from build123d import *

# Parameters (mm, degrees)
SKETCH_1_R           = 23
EXTRUDE_1_DEPTH      = 6
EXTRUDE_2_DEPTH      = 25
EXTRUDE_2_DEPTH_BACK = 9
SKETCH_2_R           = 18
SKETCH_3_R           = 10.25
CUT_EXTRUDE_1_DEPTH  = 48.053161424


with BuildPart() as part:
    # 草图1 → 凸台-拉伸1 (new body)
    with BuildSketch(Plane(origin=(0, 0, 0), x_dir=(0, 0, -1), z_dir=(1, 0, 0))):
        Circle(SKETCH_1_R)
    extrude(amount=EXTRUDE_1_DEPTH)

    # 草图2 → 凸台-拉伸2 (add, two sides: drawn at the far end of the back side and taken through both)
    with BuildSketch(Plane.ZY.offset(-EXTRUDE_2_DEPTH_BACK)):
        Circle(SKETCH_2_R)
    extrude(amount=EXTRUDE_2_DEPTH + EXTRUDE_2_DEPTH_BACK)

    # 草图3 → 切除-拉伸1 (cut, through all)
    with BuildSketch(Plane(origin=(9, 0, 0), x_dir=(0, 0, -1), z_dir=(1, 0, 0))):
        Circle(SKETCH_3_R)
    extrude(amount=-CUT_EXTRUDE_1_DEPTH, mode=Mode.SUBTRACT)


solid = part.part
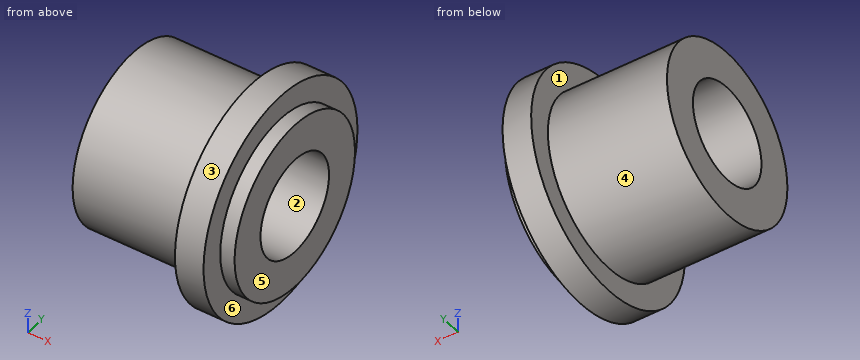
The model under review builds one solid part; all positions refer to its coordinate system, in mm. Face numbers are marked on the shaded views. A direction names the side the tool comes from. Round coordinates to 2 decimals unless told otherwise and drop trailing zeros. Loops run counter-clockwise (first coordinate to the right, second up) from the corner with the lowest first, then second, coordinate; pieces in that order, holes last. Notation, with made-up numbers: M 60.25,7.25 L 97.25,7.25 A29 cw 97.25,35.25 Z; hole C 85,0 d11. An arc over 180 degrees is marked long. Answer as CSV lines item,"result".
1. Insertion check: pin 1 Ø1.5 at (x, z) = (-16.5, -2.5) entering from -Y; pin 2 Ø4 at (y, z) = (-16.5, 11.5) entering from -X; pin 3 Ø6 at (x, z) = (-6.5, 4) entering from -Y. Each pin has a flat end and moves straight along its axis. Give the tip position at first contact, or say it passes through.
Outcome:
pin 1,"stops at y = -17.91"
pin 2,"stops at x = 0"
pin 3,"stops at y = -17.97"
2. Draft analysis for pull direction Y (two halves, no side actions). For the marked faces 1, 2 and 3, state which applies: pulls with the +Y half, pulls with the -Y half, needs draft (parallel to the pull), parting line crosses it, or undercut.
Outcome:
face 1,"needs draft"
face 2,"undercut"
face 3,"parting line crosses it"
3. For the marked faces 4, 5 and 6, list the 3-axis set-ups (+Z, -Z, +X, -X, +Y, -Y) from which the entire face can be reached by the end or side of a thin tool; tool diameter is ignored.
Outcome:
face 4,"-X"
face 5,"+Z, -Z, +X, +Y, -Y"
face 6,"+X"
4. We need section C-C (x = -4.5). Give the boundary of the cut face in (y, z), plus the area to 3 significant figures.
Outcome:
outline,"C 0,0 d36; hole C 0,0 d20.5"
area,"688 mm2"
5. We need section D-D (z = -15). Give the boundary of the cut face in (x, y).
Outcome:
outline,"M -25,-9.95 L 0,-9.95 L 0,-17.44 L 6,-17.44 L 6,-9.95 L 9,-9.95 L 9,9.95 L 6,9.95 L 6,17.44 L 0,17.44 L 0,9.95 L -25,9.95 Z"
6. To check wall thickness, follow L1, parallel to Y at x = -16.5, z = 0; L2, parallel to X at y = -6, z = 18; L3, parallel to Y at x = 3.5, z = 1.5. State the ranges of each line that lie inside material, in increasing order. Write a range as [from, to].
Outcome:
L1,"y = [-18, -10.25], [10.25, 18]"
L2,"x = [0, 6]"
L3,"y = [-22.95, -10.14], [10.14, 22.95]"
7. We need section A-A (y = 0). Give the boundary of the cut face in (x, z).
Outcome:
outline,"M -25,-18 L 0,-18 L 0,-23 L 6,-23 L 6,-18 L 9,-18 L 9,-10.25 L -25,-10.25 Z; M -25,10.25 L 9,10.25 L 9,18 L 6,18 L 6,23 L 0,23 L 0,18 L -25,18 Z"
